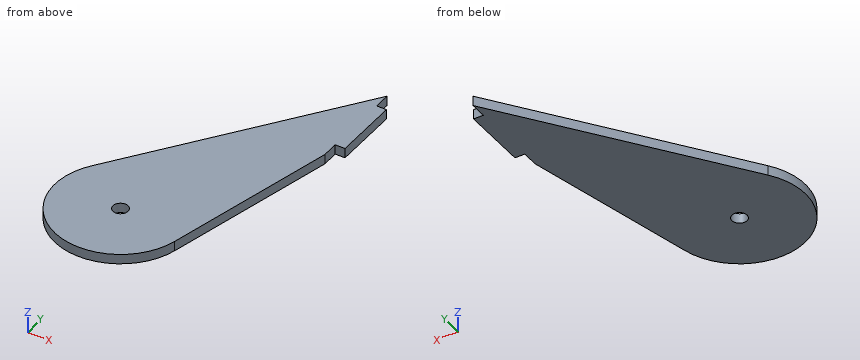
from build123d import *

# Parameters (mm, degrees)
BOSS_EXTRUDE1_DEPTH = 3
SKETCH2_R           = 2.3
CUT_EXTRUDE1_DEPTH  = 10
SKETCH4_W           = 3
SKETCH4_H           = 20
BOSS_EXTRUDE3_DEPTH = 3


with BuildPart() as part:
    # Sketch1 → Boss-Extrude1 (new body)
    with BuildSketch(Plane.XY):
        with BuildLine():
            Line((-16.174411119, 11.763860972), (32, 78))
            Line((32, 78), (32, 48))
            Line((32, 48), (19.455095298, -4.636730199))
            ThreePointArc((19.455095298, -4.636730199), (-8.362748941, -18.167675419), (-16.174411119, 11.763860972))
        make_face()
    extrude(amount=-BOSS_EXTRUDE1_DEPTH)

    # Sketch2 → Cut-Extrude1 (cut)
    with BuildSketch(Plane.XY):
        Circle(SKETCH2_R)
    extrude(amount=-CUT_EXTRUDE1_DEPTH, mode=Mode.SUBTRACT)

    # Sketch4 → Boss-Extrude3 (add)
    with BuildSketch(Plane(origin=(32, 0, 0), x_dir=(0, 0, -1), z_dir=(1, 0, 0))):
        with Locations((1.5, 63)):
            Rectangle(SKETCH4_W, SKETCH4_H)
    extrude(amount=BOSS_EXTRUDE3_DEPTH)


solid = part.part
Build history of the part. All positions in model axes, mm. Give positions to 0.01 mm unless a question says otherwise; leave off trailing zeros. Order: outer loops, then holes, each group sorted by start corner. A loop starts at its lowest first (then second) coordinate and runs counter-clockwise, first axis right, second up. Notation, with made-up numbers: M 52,8 L 71,8 A14 cw 71,14 Z; hole C 62,31 d10. An arc over 180 degrees is marked long. Put each result on its own line as item: value.
Item 1: Cut at A-A on x = 0. Write the cut outline in (y, z).
Results are:
outline: M -20,-3 L -2.3,-3 L -2.3,0 L -20,0 Z; M 2.3,-3 L 34,-3 L 34,0 L 2.3,0 Z
Item 2: Cut at D-D on y = 57.5. Write the cut outline in (x, z), then the cut area to 3 significant figures.
Results are:
outline: M 17.09,-3 L 35,-3 L 35,0 L 17.09,0 Z
area: 53.7 mm2
Item 3: Cut at B-B on z = -2. Write the cut outline in (x, y), then the cut area to 3 significant figures.
Results are:
outline: M -16.17,11.76 A20 ccw long 19.46,-4.64 L 32,48 L 32,53 L 35,53 L 35,73 L 32,73 L 32,78 Z; hole C 0,0 d4.6
area: 2,590 mm2
Item 4: Cut at C-C on y = 0. Write the cut outline in (x, z).
Results are:
outline: M -20,-3 L -2.3,-3 L -2.3,0 L -20,0 Z; M 2.3,-3 L 20.56,-3 L 20.56,0 L 2.3,0 Z
Item 5: Wall check: probe 1 along Y at (x, z) = (0, -0.9); probe 2 along X at (y, z) = (-2, -0.15); probe 3 along X at (y, z) = (60, -0.9). Give the ranges that are in metal, low to high.
Results are:
probe 1: -20 to -2.3, 2.3 to 34
probe 2: -19.9 to -1.14, 1.14 to 20.08
probe 3: 18.91 to 35
Item 6: Drop flat-ended pins along their axis: pin 1 Ø5 at (x, y) = (15, 1) entering from +Z; pin 2 Ø1.5 at (x, z) = (19.5, -2) entering from +Y; pin 3 Ø1.5 at (x, z) = (33, -1.5) entering from +Y. Give the stop position or say it passes through.
Results are:
pin 1: z = 0
pin 2: y = 61.84
pin 3: y = 73
